Part model, mm, in its own coordinate system. A direction names the side the tool comes from. Coordinates: 2 decimals unless noted, no trailing zeros. Write each loop counter-clockwise with the first axis right and the second up, starting at its lowest first coordinate (ties: lowest second). Pieces come first, ordered by that corner, then holes. Notation, with made-up numbers: M -14.75,-13 L 37.25,-13 A26 cw 37.25,14 Z; hole C 58,31 d1. An arc over 180 degrees is marked long. Use a Markdown table: item, result. Add a question column.
Q1. Slice it at C-C on x = 10.5. Write the cut outline in (y, z), then the cut area to 3 significant figures.
Q2. Pin check, flat tips, straight feed: pin 1 Ø1.7 at (y, z) = (9, 0) entering from +X; pin 2 Ø12 at (x, z) = (-14.5, 39.5) entering from +Y; pin 3 Ø2.5 at (y, z) = (5.5, -8.5) entering from -X. Stop position of each tip, or through.
Q3. Slice it at D-D on y = 4.5. Write the cut outline in (x, z), then the cut area to 3 significant figures.
Q4. Tool access for faces 5 (the cylindrical face through (-46.31, 0.23, 13.75)), 6 (the flat face through (-49, 0, 0)), 7 (the flat face through (44, -11, 5)): list every direction of +Z, -Z, +X, -X, +Y, -Y with a clear straight run to the whole face (end or side of a thin tool).
Q5. Slice it at B-B on y = 18.5. Write the cut outline in (x, z), then the cut area to 3 significant figures.
Q6. Slice it at A-A on z = 0. Write the cut outline in (x, y).
Q7. Wall check: L1, parallel to Z at x = 31.5, y = 35; L2, parallel to X at y = 30, z = -10; L3, parallel to Z at x = -13, y = -22.5. Give the ranges that are in metal, low to high. Write a range as from..to.
Q8. Mould opens along X. For faces 1 (the flat face through (-44.5, -0.2, -10.3)), 2 (the cylindrical face through (-47.986, 7.493, 0.33)), 3 (the flat face through (-44.5, 8, 0)), 4 (the flat face through (-44.5, -8, 0)) say: released by +X, released by -X, zero draft, split by the parting line, or undercut.
from build123d import *

# Parameters (mm, degrees)
F2_R      = 50
F2_R_2    = 45
F3_DEPTH  = 5
F5_R      = 13.75
F6_DEPTH  = 5.5
F7_R      = 10
F8_DEPTH  = 2.5
F9_R      = 7.5
F10_DEPTH = 2


with BuildPart() as f1:
    # F0 (on Front) → F1 (revolve)
    with BuildSketch(Plane.XZ):
        with BuildLine():
            Line((0, 50), (0, -50))
            ThreePointArc((0, -50), (50, 0), (0, 50))
        make_face()
    revolve(axis=Axis((0, 0, 0), (0, 0, -1)))

    # F2 (on Top) → F3 (cut, symmetric)
    with BuildSketch(Plane.XY):
        Circle(F2_R)
        Circle(F2_R_2, mode=Mode.SUBTRACT)
    extrude(amount=F3_DEPTH, both=True, mode=Mode.SUBTRACT)

    # F5 (on offset) → F6 (cut)
    with BuildSketch(Plane.YZ.offset(-50)):
        Circle(F5_R)
    extrude(amount=F6_DEPTH, mode=Mode.SUBTRACT)

    # F7 (on face) → F8 (join)
    with BuildSketch(Plane(origin=(-44.5, 0, 0), x_dir=(0, -1, 0), z_dir=(-1, 0, 0))):
        Circle(F7_R)
    extrude(amount=F8_DEPTH)

    # F9 (on face) → F10 (join)
    with BuildSketch(Plane(origin=(-47, 0, 0), x_dir=(0, -1, 0), z_dir=(-1, 0, 0))):
        Circle(F9_R)
    extrude(amount=F10_DEPTH)


solid = f1.part
Recorded:
| question | item | result |
|---|---|---|
| 1 | outline | M -48.63,-5 A48.89 ccw 48.63,-5 L 43.76,-5 L 43.76,5 L 48.63,5 A48.89 ccw -48.63,5 L -43.76,5 L -43.76,-5 Z |
| 1 | area | 7,410 mm² |
| 2 | pin 1 | x = 44.26 |
| 2 | pin 2 | y = 34.62 |
| 2 | pin 3 | x = -47 |
| 3 | outline | M -49,-6 L -47,-6 L -47,-8.93 L -44.5,-8.93 L -44.5,-12.99 L -48.07,-12.99 A49.8 ccw 49.55,-5 L 44.77,-5 L 44.77,5 L 49.55,5 A49.8 ccw -48.07,12.99 L -44.5,12.99 L -44.5,8.93 L -47,8.93 L -47,6 L -49,6 Z |
| 3 | area | 7,690 mm² |
| 4 | face 5 | -X |
| 4 | face 6 | +Z, -Z, -X, +Y, -Y |
| 4 | face 7 | none |
| 5 | outline | M -46.18,-5 A46.45 ccw 46.18,-5 L 41.02,-5 L 41.02,5 L 46.18,5 A46.45 ccw -46.18,5 L -41.02,5 L -41.02,-5 Z |
| 5 | area | 6,670 mm² |
| 6 | outline | M -49,-7.5 L -47,-7.5 L -47,-10 L -44.5,-10 L -44.5,-6.69 A45 ccw long -44.5,6.69 L -44.5,10 L -47,10 L -47,7.5 L -49,7.5 Z |
| 7 | L1 | -16.82..-5, 5..16.82 |
| 7 | L2 | -38.73..38.73 |
| 7 | L3 | -42.72..42.72 |
| 8 | face 1 | released by -X |
| 8 | face 2 | zero draft |
| 8 | face 3 | undercut |
| 8 | face 4 | undercut |
